For this review, take the finished solid that the model builds, in its own axes (mm). A direction names the side the tool comes from. Give positions to 0.01 mm unless a question says otherwise; leave off trailing zeros. Loops run counter-clockwise (first coordinate to the right, second up) from the corner with the lowest first, then second, coordinate; pieces in that order, holes last. Notation, with made-up numbers: (8, -25.75) - (28, -25.75) arc R23 ccw to (28, -6.75) - close; hole circle Ø1 at (24, -10). An arc over 180 degrees is marked (long way). Put each result on its own line as item: value.
Autodesk Inventor part; units mm, degrees
ref_plane "YZ Plane" through (0, 0, 0) normal (1, 0, 0) x (0, 1, 0)
ref_plane "XZ Plane" through (0, 0, 0) normal (0, 1, 0) x (-1, 0, 0)
ref_plane "XY Plane" through (0, 0, 0) normal (0, 0, 1) x (1, 0, 0)
sketch "Sketch1" plane through (0, 0, 0) normal (0, 1, 0) x (-1, 0, 0)
  line L0 (-613.8, 55) -> (-513.8, 55)
  line L1 (-387.5, 55) -> (-613.8, 55)
  line L2 (-513.8, 55) -> (-473.8, 55)
  line L3 (-469.3, 380.5) -> (-343, 380.5)
  line L4 (-343, 390.5) -> (-469.3, 390.5)
  line L5 (-474.3, 385.5) -> (-474.3, 385.5)
  circle A0 centre (-658.3, 385.5) radius 5
  arc A1 (-474.3, 385.5) -> (-469.3, 380.5) centre (-469.3, 385.5) ccw
  arc A2 (-469.3, 390.5) -> (-474.3, 385.5) centre (-469.3, 385.5) ccw
  line L6 (-513.8, 395) -> (-513.8, 395.5)
  line L7 (-513.8, 55) -> (-469.3, 55)
  line L8 (-474.3, 65) -> (-474.3, 65)
  line L9 (-474.3, 178.5) -> (-474.3, 178.5)
  line L10 (-474.3, 292) -> (-474.3, 292)
  line L11 (-653.3, 45) -> (-653.3, 272)
  line L12 (-663.3, 45) -> (-663.3, 272)
  line L13 (-613.8, 395.5) -> (-513.8, 395.5)
  line L14 (-513.8, 395.5) -> (-513.8, 168.5)
  line L15 (-513.8, 168.5) -> (-613.8, 168.5)
  line L16 (-513.8, 168.5) -> (-387.5, 168.5)
  line L17 (-613.8, 168.5) -> (-613.8, 395.5)
  line L18 (-513.8, 395.5) -> (-513.8, 29.6)
  line L19 (-613.8, 29.6) -> (-613.8, 168.5)
  line L20 (-387.5, 29.6) -> (-387.5, 395.5)
  line L21 (-387.5, 395.5) -> (-513.8, 395.5)
  line L22 (-387.5, 29.6) -> (-613.8, 29.6)
  line L23 (-513.8, 282) -> (-613.8, 282)
  line L24 (-663.3, 45) -> (-663.3, 39.6)
  line L25 (-653.3, 39.6) -> (-653.3, 45)
  arc A3 (-663.3, 39.6) -> (-653.3, 39.6) centre (-658.3, 39.6) ccw
  line L26 (-663.3, 272) -> (-663.3, 292)
  line L27 (-653.3, 292) -> (-653.3, 272)
  arc A4 (-653.3, 292) -> (-663.3, 292) centre (-658.3, 292) ccw
  line L28 (-464.3, 292) -> (-464.3, 183.5)
  line L29 (-474.3, 178.5) -> (-474.3, 292)
  arc A5 (-464.3, 292) -> (-474.3, 292) centre (-469.3, 292) ccw
  line L30 (-474.3, 183.5) -> (-474.3, 65)
  line L31 (-464.3, 70) -> (-464.3, 292)
  arc A6 (-343, 34.6) -> (-343, 44.6) centre (-343, 39.6) ccw
  line L32 (-343, 34.6) -> (-369.3, 34.6)
  line L33 (-364.3, 44.6) -> (-343, 44.6)
  line L34 (-369.3, 34.6) -> (-364.3, 34.6)
  line L35 (-663.3, 183.5) -> (-676.3, 183.5)
  line L36 (-676.3, 6.6) -> (-676.3, 418.5)
  line L37 (-324.4347, 22.1004) -> (-324.4347, 40.1004)
  line L38 (-324.4127, 6.6) -> (-324.9989, 418.5)
  arc A7 (-343, 380.5) -> (-343, 390.5) centre (-343, 385.5) ccw
  line L39 (-613.8, 55) -> (-613.8, 395.5)
  line L40 (-474.3, 65) -> (-474.3, 39.6)
  line L41 (-469.3, 34.6) -> (-369.3, 34.6)
  line L42 (-464.3, 70) -> (-464.3, 44.6)
  line L43 (-464.3, 44.6) -> (-364.3, 44.6)
  arc A8 (-474.3, 39.6) -> (-469.3, 34.6) centre (-469.3, 39.6) ccw
  line L44 (-437.15, 411.5) -> (-564.15, 411.5)
  line L45 (-437.15, 13.6) -> (-564.15, 13.6)
  line L46 (-324.4127, 6.6) -> (-676.3, 6.6)
  line L47 (-676.3, 418.5) -> (-324.9989, 418.5)
  point P0 (-469.3, 178.5)
  point P1 (-469.3, 292)
  point P2 (-474.3, 385.5)
  dimension "d9" = 10
  dimension "d75" = 126.3
  dimension "d76" = 226.3
  dimension "d78" = 10
  dimension "d79" = 10
  dimension "d82" = 10
  dimension "d92" = 10
  dimension "d98" = 13
  dimension "d205" = 365.9
  dimension "d206" = 227
  dimension "d207" = 340.5
  dimension "d208" = 5
  dimension "d238" = 127
  dimension "d240" = 127
extrude "Extrusion1" add sketch "Sketch1" along normal blind 3.175 contours L19 L15 L18 L0 | L0 L18 L22 L19 | L18 L16 L30 L40 L1 | L1 L40 A8 L41 L20 L22 L18 | L17 L23 L14 L15 | L14 L6 L21 L20 L4 A2 A1 L3 L16 L31 L28 A5 L29 L30 | L17 L13 L6 L14 L23 | L16 L20 L1 L42 L31 | L1 L20 L43 L42 | L36 L47 L38 L46
sketch "Sketch2" plane through (0, 0, 0) normal (0, -1, 0) x (1, 0, 0)
  line L0 (474.3, 178.5) -> (474.3, 178.5)
  line L1 (513.8, 168.5) -> (413.8, 168.5)
  line L2 (413.8, 395.5) -> (413.8, 55)
  line L3 (513.8, 395.5) -> (513.8, 29.6)
  line L4 (387.5, 29.6) -> (387.5, 395.5)
  line L5 (474.3, 65) -> (474.3, 65)
  line L6 (474.3, 385.5) -> (474.3, 385.5)
  line L7 (513.8, 395) -> (513.8, 395.5)
  line L8 (613.8, 29.6) -> (613.8, 168.5)
  line L9 (613.8, 55) -> (513.8, 55)
  line L10 (513.8, 55) -> (473.8, 55)
  line L11 (513.8, 55) -> (469.3, 55)
  line L12 (413.8, 55) -> (613.8, 55)
  line L13 (613.8, 168.5) -> (613.8, 395.5)
  line L14 (513.8, 395.5) -> (513.8, 168.5)
  line L15 (513.8, 168.5) -> (613.8, 168.5)
  line L16 (474.3, 292) -> (474.3, 292)
  line L17 (387.5, 29.6) -> (613.8, 29.6)
  line L18 (513.8, 282) -> (613.8, 282)
  line L19 (387.5, 395.5) -> (513.8, 395.5)
  line L20 (613.8, 395.5) -> (513.8, 395.5)
  line L21 (475.3, 378.5) -> (337, 378.5)
  line L22 (337, 392.5) -> (475.3, 392.5)
  circle A0 centre (658.3, 385.5) radius 7.75
  line L23 (665.3, 272) -> (665.3, 298)
  line L24 (651.3, 298) -> (651.3, 272)
  line L25 (651.3, 272) -> (651.3, 45)
  line L26 (651.3, 45) -> (651.3, 33.6)
  line L27 (665.3, 33.6) -> (665.3, 45)
  line L28 (665.3, 45) -> (665.3, 272)
  line L29 (369.3, 32.6) -> (337, 32.6)
  line L30 (337, 46.6) -> (355.3, 46.6)
  line L31 (462.3, 79) -> (462.3, 164.5)
  line L32 (462.3, 192.5) -> (462.3, 298)
  line L33 (476.3, 65) -> (476.3, 183.5)
  line L34 (476.3, 178.5) -> (476.3, 298)
  arc A1 (476.3, 298) -> (462.3, 298) centre (469.3, 298) ccw
  arc A2 (337, 46.6) -> (337, 32.6) centre (337, 39.6) ccw
  arc A3 (651.3, 33.6) -> (665.3, 33.6) centre (658.3, 33.6) ccw
  arc A4 (665.3, 298) -> (651.3, 298) centre (658.3, 298) ccw
  arc A5 (475.3, 378.5) -> (475.3, 392.5) centre (475.3, 385.5) ccw
  arc A6 (337, 392.5) -> (337, 378.5) centre (337, 385.5) ccw
  line L35 (476.3, 65) -> (476.3, 39.6)
  line L36 (469.3, 32.6) -> (369.3, 32.6)
  line L37 (343, 34.6) -> (469.3, 34.6)
  line L38 (462.3, 79) -> (462.3, 53.6)
  line L39 (464.3, 44.6) -> (343, 44.6)
  line L40 (455.3, 46.6) -> (355.3, 46.6)
  arc A7 (469.3, 32.6) -> (476.3, 39.6) centre (469.3, 39.6) ccw
  arc A8 (455.3, 46.6) -> (462.3, 53.6) centre (455.3, 53.6) ccw
  line L41 (462.3, 164.5) -> (462.3, 192.5)
  line L42 (464.3, 292) -> (464.3, 44.6)
  line L43 (676.3, 11.6) -> (324.4127, 11.6)
  line L44 (324.4127, 6.6) -> (324.9989, 418.5)
  line L45 (325, 413.5) -> (676.3, 413.5)
  line L46 (676.3, 418.5) -> (676.3, 6.6)
  point P0 (650, 0)
  point P1 (0, 41.6)
  point P2 (0, 378.5)
  point P3 (413.8, 282)
  point P4 (469.3, 178.5)
  point P5 (676.3, 450)
  point P6 (676.3, 0)
  point P7 (513.8, 55)
  point P8 (513.8, 29.6)
  point P9 (362.3, 46.6)
  point P10 (462.3, 72)
  point P11 (462.3, 171.5)
  point P12 (462.3, 185.5)
  point P13 (376.3, 58)
  point P14 (325, 424)
  point P15 (324.9989, 418.5)
  dimension "d178" = 15.5
  dimension "d186" = 14
  dimension "d190" = 14
  dimension "d192" = 14
  dimension "d194" = 14
  dimension "d198" = 14
  dimension "d202" = 14
  dimension "d209" = 7
extrude "Extrusion2" cut sketch "Sketch2" against normal blind 2 contours L33 L35 L10 L11 L12 L42 L1 | L1 L41 L32 A1 L34 L33 | L42 L12 L38 L31 L41 L1 | L35 A7 L36 L4 L39 L42 L12 L11 L10 | L42 L39 L4 L40 A8 L38 L12 | L36 L29 A2 L30 L40 L4 | L21 L4 L22 L2 | L2 L22 A5 L21 | L21 A6 L22 L4 | A0 | L28 L27 A3 L26 L25 L24 A4 L23
fillet "Fillet1" radius 20 4 edges at (324.4127, 1.5875, 6.6) (676.3, 1.5875, 6.6) (676.3, 1.5875, 418.5) (324.9989, 1.5875, 418.5)
hole "Hole2" at (437.15, 0, 13.6) at (564.15, 0, 13.6) at (437.15, 0, 411.5) at (564.15, 0, 411.5) direction (0, 1, 0) diameter 8 end through all counterbore diameter 12 counterbore depth 2
properties part number "PlateLateral" material "Aluminum, Anodized Silver"
1) For faces 1 (the face through (406, 2, 391)), 2 (the face through (330.684, 1.61, 412.496)), list the 3-axis set-ups (+Z, -Z, +X, -X, +Y, -Y) from which the entire face can be reached by the end or side of a thin tool; tool diameter is ignored.
Geometry check:
face 1: -Y
face 2: +Z, -X, +Y, -Y
2) Take a section at A-A on y = 2.65. State how many separate pieces and enclosed holes the cut face has, and give its area (3 significant figures).
Geometry check:
separate pieces: 1
enclosed holes: 8
area: 136,000 mm²
3) Take a section at C-C on z = 385.5. State the section outline as (x, y) points (3 decimals), and give its area (3 significant figures).
Geometry check:
outline: (324.952, 0) - (330, 0) - (330, 2) - (338, 2) - (338, 3.175) - (324.952, 3.175) - close; (474.3, 2) - (482.3, 2) - (482.3, 0) - (650.55, 0) - (650.55, 2) - (653.3, 2) - (653.3, 3.175) - (474.3, 3.175) - close; (663.3, 2) - (666.05, 2) - (666.05, 0) - (676.3, 0) - (676.3, 3.175) - (663.3, 3.175) - close
area: 608 mm²
4) Take a section at B-B on z = 264. State the section outline as (x, y) points (3 decimals), and give its area (3 significant figures).
Geometry check:
outline: (324.779, 0) - (462.3, 0) - (462.3, 2) - (464.3, 2) - (464.3, 3.175) - (324.779, 3.175) - close; (474.3, 2) - (476.3, 2) - (476.3, 0) - (651.3, 0) - (651.3, 2) - (653.3, 2) - (653.3, 3.175) - (474.3, 3.175) - close; (663.3, 2) - (665.3, 2) - (665.3, 0) - (676.3, 0) - (676.3, 3.175) - (663.3, 3.175) - close
area: 1,040 mm²
5) Draft analysis for pull direction X (two halves, no side actions). For faces 3 (the face through (661.876, 0.986, 378.624)), 4 (the face through (670.597, 1.61, 12.614)), 5 (the face through (503, 3.175, 215)), state which applies: pulls with the +X half, pulls with the -X half, needs draft (parallel to the pull), parting line crosses it, or undercut.
Geometry check:
face 3: undercut
face 4: pulls with the +X half
face 5: needs draft
6) Wall thickness on line 1 (Z direction, x = 426, y = 1.55); line 2 (Z direction, x = 564.15, y = 2.8); line 3 (Z direction, x = 437.15, y = 2.4): over which ranges is each line inside the solid? List them lowest first.
Geometry check:
line 1: z = 6.6 to 32.6, 46.6 to 378.5, 392.5 to 418.5
line 2: z = 6.6 to 9.6, 17.6 to 407.5, 415.5 to 418.5
line 3: z = 6.6 to 9.6, 17.6 to 34.6, 44.6 to 380.5, 390.5 to 407.5, 415.5 to 418.5
7) Insertion check: pin 1 Ø7 at (x, z) = (437.15, 411.5) entering from -Y; pin 2 Ø1.3 at (y, z) = (2.5, 216.5) entering from -X. Each pin has a flat end and moves straight along its axis. Give the tip position at first contact, or say it passes through.
Geometry check:
pin 1: passes through
pin 2: stops at x = 324.71
